```python
from build123d import *

# Parameters (mm, degrees)
SKETCH1_W           = 35
SKETCH1_H           = 35
BOSS_EXTRUDE1_DEPTH = 27
SHELL1_T            = -2
CUT_EXTRUDE7_DEPTH  = 33
BOSS_EXTRUDE4_DEPTH = 31
BOSS_EXTRUDE3_DEPTH = 26
FILLET1_R           = 1
FILLET2_R           = 1
FILLET3_R           = 1
FILLET4_R           = 1
SKETCH10_R          = 1.65
CUT_EXTRUDE3_DEPTH  = 36.178118199
SKETCH11_W          = 16
SKETCH11_H          = 9
CUT_EXTRUDE4_DEPTH  = 2
SKETCH13_R          = 2.6
CUT_EXTRUDE6_DEPTH  = 2
FILLET5_R           = 3
FILLET6_R           = 1


with BuildPart() as part:
    # Sketch1 → Boss-Extrude1 (new body)
    with BuildSketch(Plane(origin=(0, 0, 0), x_dir=(1, 0, 0), z_dir=(0, 1, 0))):
        Rectangle(SKETCH1_W, SKETCH1_H)
    extrude(amount=BOSS_EXTRUDE1_DEPTH)

    # Shell1
    shell1_openings = [part.faces().sort_by_distance(p)[0] for p in [
        (0, 27, 0),
    ]]
    offset(amount=SHELL1_T, openings=shell1_openings, kind=Kind.INTERSECTION)

    # Sketch5 → Cut-Extrude7 (cut)
    with BuildSketch(Plane.XY.offset(17.5)):
        Polygon((-12.412133126, 27), (12.412133126, 27), (14.912133126, 24.5), (-14.912133126, 24.5), align=None)
    extrude(amount=-CUT_EXTRUDE7_DEPTH, mode=Mode.SUBTRACT)

    # Sketch16 → Boss-Extrude4 (add)
    with BuildSketch(Plane(origin=(0, 0, 15.5), x_dir=(-1, 0, 0), z_dir=(0, 0, -1))):
        Polygon((-15.5, 27), (-12.412133126, 27), (-14.912133126, 24.5), (-13.5, 24.5), (-13.5, 22.5), (-15.5, 22.5), align=None)
        Polygon((13.5, 22.5), (15.5, 22.5), (15.5, 27), (12.412133126, 27), (14.912133126, 24.5), (13.5, 24.5), align=None)
    extrude(amount=BOSS_EXTRUDE4_DEPTH)

    # Sketch9 → Boss-Extrude3 (add)
    with BuildSketch(Plane.XY.offset(17.5)):
        Polygon((-9.517157288, 0), (-12.517157288, -3), (12.517157288, -3), (9.517157288, 0), align=None)
    extrude(amount=-BOSS_EXTRUDE3_DEPTH)

    # Fillet1
    fillet1_edges = [part.edges().sort_by_distance(p)[0] for p in [
        (15.5, 2, 0),
        (0, 2, -15.5),
        (-15.5, 2, 0),
        (0, 2, 15.5),
        (15.5, 12.25, 15.5),
        (15.5, 12.25, -15.5),
        (-15.5, 12.25, -15.5),
        (-15.5, 12.25, 15.5),
    ]]
    fillet(fillet1_edges, radius=FILLET1_R)

    # Fillet2
    fillet2_edges = [part.edges().sort_by_distance(p)[0] for p in [
        (-17.5, 27, 0),
        (17.5, 27, 0),
        (-17.5, 0, 0),
        (17.5, 0, 0),
        (17.5, 13.5, 17.5),
        (-17.5, 13.5, 17.5),
        (-17.5, 13.5, -17.5),
        (17.5, 13.5, -17.5),
    ]]
    fillet(fillet2_edges, radius=FILLET2_R)

    # Fillet3
    # the kernel refuses this fillet: 1 mm, written as the material it takes off along each edge
    with BuildSketch(Plane(origin=(16.5, 26, -16.5), x_dir=(0, 0, -1), z_dir=(0, 1, 0))) as fillet3_piece_1_section:
        Polygon((0, 0), (FILLET3_R, 0), (FILLET3_R, -FILLET3_R), (0, -FILLET3_R), align=None)
    fillet3_piece_1 = extrude(amount=FILLET3_R, mode=Mode.PRIVATE)
    fillet3_piece_1 = fillet3_piece_1 - Plane(origin=(16.5, 26, -16.5), x_dir=(-0.7071067811865475, 0, 0.7071067811865475), z_dir=(0, 1, 0)) * Sphere(FILLET3_R, mode=Mode.PRIVATE)
    add(fillet3_piece_1, mode=Mode.SUBTRACT)
    with BuildSketch(Plane(origin=(16.5, 1, -16.5), x_dir=(0, -1, 0), z_dir=(0, 0, -1))) as fillet3_piece_2_section:
        Polygon((0, 0), (FILLET3_R, 0), (FILLET3_R, -FILLET3_R), (0, -FILLET3_R), align=None)
    fillet3_piece_2 = extrude(amount=FILLET3_R, mode=Mode.PRIVATE)
    fillet3_piece_2 = fillet3_piece_2 - Plane(origin=(16.5, 1, -16.5), x_dir=(-0.7071067811865475, 0.7071067811865475, 0), z_dir=(0, 0, -1)) * Sphere(FILLET3_R, mode=Mode.PRIVATE)
    add(fillet3_piece_2, mode=Mode.SUBTRACT)
    with BuildSketch(Plane(origin=(-16.5, 26, -16.5), x_dir=(0, 0, -1), z_dir=(0, 1, 0))) as fillet3_piece_3_section:
        Polygon((0, 0), (FILLET3_R, 0), (FILLET3_R, FILLET3_R), (0, FILLET3_R), align=None)
    fillet3_piece_3 = extrude(amount=FILLET3_R, mode=Mode.PRIVATE)
    fillet3_piece_3 = fillet3_piece_3 - Plane(origin=(-16.5, 26, -16.5), x_dir=(0.7071067811865475, 0, 0.7071067811865475), z_dir=(0, 1, 0)) * Sphere(FILLET3_R, mode=Mode.PRIVATE)
    add(fillet3_piece_3, mode=Mode.SUBTRACT)
    with BuildSketch(Plane(origin=(-16.5, 1, -16.5), x_dir=(0, -1, 0), z_dir=(0, 0, -1))) as fillet3_piece_4_section:
        Polygon((0, 0), (FILLET3_R, 0), (FILLET3_R, FILLET3_R), (0, FILLET3_R), align=None)
    fillet3_piece_4 = extrude(amount=FILLET3_R, mode=Mode.PRIVATE)
    fillet3_piece_4 = fillet3_piece_4 - Plane(origin=(-16.5, 1, -16.5), x_dir=(0.7071067811865475, 0.7071067811865475, 0), z_dir=(0, 0, -1)) * Sphere(FILLET3_R, mode=Mode.PRIVATE)
    add(fillet3_piece_4, mode=Mode.SUBTRACT)
    with BuildSketch(Plane(origin=(16.5, 27, -17.5), x_dir=(0, 0, 1), z_dir=(-1, 0, 0)), Plane(origin=(16.5, 0, -17.5), x_dir=(0, 1, 0), z_dir=(-1, 0, 0))) as fillet3_piece_5:
        with BuildLine():
            CenterArc((FILLET3_R, -FILLET3_R), FILLET3_R, 90, 90)
            Line((0, -FILLET3_R), (0, 0))
            Line((0, 0), (FILLET3_R, 0))
        make_face()
    extrude(amount=33, mode=Mode.SUBTRACT)

    # Fillet4
    # the kernel refuses this fillet: 1 mm, written as the material it takes off along each edge
    with BuildSketch(Plane(origin=(16.5, 26, 16.5), x_dir=(0, 0, 1), z_dir=(0, 1, 0))) as fillet4_piece_1_section:
        Polygon((0, 0), (FILLET4_R, 0), (FILLET4_R, FILLET4_R), (0, FILLET4_R), align=None)
    fillet4_piece_1 = extrude(amount=FILLET4_R, mode=Mode.PRIVATE)
    fillet4_piece_1 = fillet4_piece_1 - Plane(origin=(16.5, 26, 16.5), x_dir=(-0.7071067811865475, 0, -0.7071067811865475), z_dir=(0, 1, 0)) * Sphere(FILLET4_R, mode=Mode.PRIVATE)
    add(fillet4_piece_1, mode=Mode.SUBTRACT)
    with BuildSketch(Plane(origin=(-16.5, 26, 16.5), x_dir=(0, 0, 1), z_dir=(0, 1, 0))) as fillet4_piece_2_section:
        Polygon((0, 0), (FILLET4_R, 0), (FILLET4_R, -FILLET4_R), (0, -FILLET4_R), align=None)
    fillet4_piece_2 = extrude(amount=FILLET4_R, mode=Mode.PRIVATE)
    fillet4_piece_2 = fillet4_piece_2 - Plane(origin=(-16.5, 26, 16.5), x_dir=(0.7071067811865475, 0, -0.7071067811865475), z_dir=(0, 1, 0)) * Sphere(FILLET4_R, mode=Mode.PRIVATE)
    add(fillet4_piece_2, mode=Mode.SUBTRACT)
    with BuildSketch(Plane(origin=(-16.5, 27, 17.5), x_dir=(0, 0, -1), z_dir=(1, 0, 0)), Plane(origin=(9.912133126, 27, 17.5), x_dir=(0, 0, -1), z_dir=(1, 0, 0))) as fillet4_piece_3:
        with BuildLine():
            CenterArc((FILLET4_R, -FILLET4_R), FILLET4_R, 90, 90)
            Line((0, -FILLET4_R), (0, 0))
            Line((0, 0), (FILLET4_R, 0))
        make_face()
    extrude(amount=6.587866874, mode=Mode.SUBTRACT)

    # Sketch10 → Cut-Extrude3 (cut, through all)
    with BuildSketch(Plane(origin=(0, 2, 0), x_dir=(1, 0, 0), z_dir=(0, 1, 0))):
        with Locations(Location((-7.5, -9.5, 0), (0, 0, 270))):
            Circle(SKETCH10_R)
        with Locations(Location((7.5, -9.5, 0), (0, 0, 270))):
            Circle(SKETCH10_R)
    extrude(amount=-CUT_EXTRUDE3_DEPTH, mode=Mode.SUBTRACT)

    # Sketch11 → Cut-Extrude4 (cut)
    with BuildSketch(Plane(origin=(0, 0, 17.5), x_dir=(-1, 0, 0), z_dir=(0, 0, -1))):
        with Locations((0.5, 16)):
            Rectangle(SKETCH11_W, SKETCH11_H)
    extrude(amount=CUT_EXTRUDE4_DEPTH, mode=Mode.SUBTRACT)

    # Sketch13 → Cut-Extrude6 (cut)
    with BuildSketch(Plane.XZ.offset(3)):
        with Locations((-7.5, 9.5)):
            Circle(SKETCH13_R)
        with Locations((7.5, 9.5)):
            Circle(SKETCH13_R)
    extrude(amount=-CUT_EXTRUDE6_DEPTH, mode=Mode.SUBTRACT)

    # Fillet5
    fillet5_edges = [part.edges().sort_by_distance(p)[0] for p in [
        (13.5, 23.5, -15.5),
        (-13.5, 23.5, -15.5),
    ]]
    fillet(fillet5_edges, radius=FILLET5_R)

    # Fillet6
    fillet6_edges = [part.edges().sort_by_distance(p)[0] for p in [
        (-15.207106781, 22.5, -15.207106781),
        (-15.207106781, 22.5, 15.207106781),
        (15.5, 22.5, 0),
        (15.207106781, 22.5, 15.207106781),
        (15.207106781, 22.5, -15.207106781),
        (12.5, 22.5, -15.5),
        (-14, 22.5, 15.5),
        (-15.5, 22.5, 0),
        (14, 22.5, 15.5),
        (-12.5, 22.5, -15.5),
    ]]
    fillet(fillet6_edges, radius=FILLET6_R)


solid = part.part
```
CAD build for the part. Positions are in the model's coordinates, mm. A direction names the side the tool comes from. Coordinates: 2 decimals unless noted, no trailing zeros. Order: outer loops, then holes, each group sorted by start corner. A loop starts at its lowest first (then second) coordinate and runs counter-clockwise, first axis right, second up. Notation, with made-up numbers: M 41,20.5 L 60,20.5 A36 ccw 60,57.5 Z; hole C -26,-4.75 d9. An arc over 180 degrees is marked long. Write each question's results on one line, items separated by ' | '. Start each with the question number.
Q1. Cut at B-B (y = 7.5). List the corners of the cut face in (x, z).
Q2. Cut at A-A (x = -7.5). List the corners of the cut face in (y, z).
Q3. Which spindle directions (+Z, -Z, +X, -X, +Y, -Y) get a long thin tool onto all of the face, cutting with end or side? Do faces 1 (the cylindrical face through (15.215, 12.38, 15.199)), 2 (the flat face through (0, 0, -11)), 3 (the flat face through (11.038, -1.521, 4.682)). Say none if no direction does.
Q4. Cut at C-C (x = 1). List the corners of the cut face in (y, z), then the cut area to 3 significant figures.
Q5. Drill centre lines: probe 1 along X at (y, z) = (8.25, -14.5); probe 2 along X at (y, z) = (1.25, 10). Where is each one in solid material? Low to high. Write a range as from..to.
Q6. Flat gauge pins, fed straight in: P1, Ø2.5, axis at x = -7.5, z = 9.5, coming from the -Y side; P2, Ø6, axis at x = -4, y = 16, coming from the +Z side; P3, Ø0.6, axis at x = -3, z = 16, coming from the +Y side; P4, Ø4.5, axis at x = 7.5, z = 9.5, coming from the -Y side. Where does each tip first touch, or does it go through?
Q7. Cut at D-D (z = -9). List the corners of the cut face in (x, y), then the cut area to 3 significant figures.
Q8. Pull direction Z, two halves, no side cores. Call faces 4 (the cylindrical face through (15.199, 12.12, -15.215)), 5 (the flat face through (0, 11, 17.5)), 6 (the flat face through (17.5, 13, 0)), 7 (the flat face through (0, 15, -15.5)): +Z half, -Z half, draft (parallel to the pull), parting line (faces both ways), or undercut.
Found:
1) outline: M -17.5,-16.5 A1 ccw -16.5,-17.5 L 16.5,-17.5 A1 ccw 17.5,-16.5 L 17.5,16.5 A1 ccw 16.5,17.5 L -16.5,17.5 A1 ccw -17.5,16.5 Z; hole M -15.5,-14.5 A1 ccw -14.5,-15.5 L 14.5,-15.5 A1 ccw 15.5,-14.5 L 15.5,14.5 A1 ccw 14.5,15.5 L -14.5,15.5 A1 ccw -15.5,14.5 Z
2) outline: M -3,-8.5 L 0,-8.5 L 0,-16.5 A1 ccw 1,-17.5 L 26,-17.5 A1 ccw 27,-16.5 L 27,-15.5 L 3,-15.5 A1 cw 2,-14.5 L 2,7.85 L -1,7.85 L -1,6.9 L -3,6.9 Z; M -3,12.1 L -1,12.1 L -1,11.15 L 2,11.15 L 2,14.5 A1 cw 3,15.5 L 11.5,15.5 L 11.5,17.5 L -3,17.5 Z; M 20.5,15.5 L 24.5,15.5 L 24.5,17.5 L 20.5,17.5 Z
3) face 1: none | face 2: -Z | face 3: +Z, -Z, +X
4) outline: M -3,-8.5 L 0,-8.5 L 0,-16.5 A1 ccw 1,-17.5 L 26,-17.5 A1 ccw 27,-16.5 L 27,-15.5 L 3,-15.5 A1 cw 2,-14.5 L 2,14.5 A1 cw 3,15.5 L 11.5,15.5 L 11.5,17.5 L -3,17.5 Z; M 20.5,15.5 L 24.5,15.5 L 24.5,17.5 L 20.5,17.5 Z | area: 225 mm²
5) probe 1: -17.5..-15.5, 15.5..17.5 | probe 2: -17.5..-9.07, -5.93..5.93, 9.07..17.5
6) P1: through | P2: z = -15.5 | P3: y = 24.5 | P4: y = -1
7) outline: M -17.5,1 A1 ccw -16.5,0 L 16.5,0 A1 ccw 17.5,1 L 17.5,26 A1 ccw 16.5,27 L 12.41,27 L 14.91,24.5 L 13.5,24.5 L 13.5,22.5 L 14.5,22.5 A1 cw 15.5,21.5 L 15.5,3 A1 cw 14.5,2 L -14.5,2 A1 cw -15.5,3 L -15.5,21.5 A1 cw -14.5,22.5 L -13.5,22.5 L -13.5,24.5 L -14.91,24.5 L -12.41,27 L -16.5,27 A1 ccw -17.5,26 Z | area: 187 mm²
8) face 4: undercut | face 5: +Z half | face 6: draft | face 7: undercut
